Work out the finished part from the listing and answer in its coordinate system (mm). A direction names the side the tool comes from. Give positions to 0.01 mm unless a question says otherwise; leave off trailing zeros. Write each loop counter-clockwise with the first axis right and the second up, starting at its lowest first coordinate (ties: lowest second). Pieces come first, ordered by that corner, then holes. Notation, with made-up numbers: (30, 63.5) -> (65, 63.5) arc R19 ccw to (65, 92.5) -> close; hole circle Ø6 at (54.5, -26.75). An arc over 180 degrees is marked (long way). Use a Markdown table: item, result. Add a question column.
Q1. Each of these flat-tipped pins is pushed along its axis until it touches: pin 1 Ø6.5 at (x, y) = (-21, 3) entering from +Z; pin 2 Ø4 at (x, y) = (21.5, -10) entering from +Z (3 decimals). Where does it stop, or does it pass through?
Q2. Section B-B, the plane y = 0 is taken. State how many separate pieces and enclosed holes the cut face has, plus the area to 3 significant figures.
Q3. Consider line 1 (X direction, y = 0, z = 1.35); line 2 (Y direction, x = -19.05, z = 1.5); line 3 (X direction, y = 1, z = 0.65). Determine where each line is inside the solid, lowest interval first.
Q4. For faces 1 (the face through (27, 0, 1.905)), 2 (the face through (23, -3, 1.651)), 3 (the face through (-27, 0, 1.905)), determine the directions among +Z, -Z, +X, -X, +Y, -Y from which every point of the face is accessible in a straight line to the end or side of a thin tool.
Q5. Section D-D, the plane x = -27 is taken. Give the vertices of the cut face in (y, z) (3 decimals).
Q6. For a pull along Y with two mould halves and no side action, classify faces 4 (the face through (-1, 0, 0)), 5 (the face through (-14.5, 1.4, 1.3)), 6 (the face through (-1, -12.7, 1)) as pulls with the +Y half, pulls with the -Y half, needs draft (parallel to the pull), parting line crosses it, or undercut.
from build123d import *

# Parameters (mm, degrees)
SKETCH_W        = 76.2
SKETCH_H        = 25.4
SKETCH_R        = 4.7625
PAD_DEPTH       = 1.905
SKETCH001_W     = 12.7
SKETCH001_H     = 12.7
POCKET_DEPTH    = 0.254
CHAMFER_SIZE    = 1
FILLET_R        = 1
SKETCH002_W     = 20.32
SKETCH002_H     = 25.4
PAD001_DEPTH    = 0.9525
CHAMFER001_SIZE = 0.9144


with BuildPart() as part:
    # Sketch → Pad (new body)
    with BuildSketch(Plane.XY):
        Rectangle(SKETCH_W, SKETCH_H)
        with Locations((-19.05, 0)):
            Circle(SKETCH_R, mode=Mode.SUBTRACT)
        with Locations((19.05, 0)):
            Circle(SKETCH_R, mode=Mode.SUBTRACT)
    extrude(amount=PAD_DEPTH)

    # Sketch001 → Pocket (cut)
    with BuildSketch(Plane.XY.offset(1.905)):
        with Locations((-19.05, 0)):
            Rectangle(SKETCH001_W, SKETCH001_H)
        with Locations((19.05, 0)):
            Rectangle(SKETCH001_W, SKETCH001_H)
    extrude(amount=-POCKET_DEPTH, mode=Mode.SUBTRACT)

    # Chamfer
    chamfer_edges = [part.edges().sort_by_distance(p)[0] for p in [
        (14.2875, 0, 0),
        (-23.8125, 0, 0),
    ]]
    chamfer(chamfer_edges, length=CHAMFER_SIZE)

    # Fillet
    fillet_edges = [part.edges().sort_by_distance(p)[0] for p in [
        (38.1, 12.7, 0.9525),
        (38.1, -12.7, 0.9525),
        (-38.1, -12.7, 0.9525),
        (-38.1, 12.7, 0.9525),
    ]]
    fillet(fillet_edges, radius=FILLET_R)

    # Sketch002 (on Face5 of Pocket) → Pad001 (join)
    with BuildSketch(Plane.XY.offset(1.905)):
        Rectangle(SKETCH002_W, SKETCH002_H)
    extrude(amount=PAD001_DEPTH)

    # Chamfer001
    chamfer001_edges = [part.edges().sort_by_distance(p)[0] for p in [
        (0, -12.7, 2.8575),
        (-10.16, 0, 2.8575),
        (0, 12.7, 2.8575),
        (10.16, 0, 2.8575),
    ]]
    chamfer(chamfer001_edges, length=CHAMFER001_SIZE)


solid = part.part
Result set:
| question | item | result |
|---|---|---|
| 1 | pin 1 | stops at z = 1.65 |
| 1 | pin 2 | stops at z = 1.905 |
| 2 | separate pieces | 3 |
| 2 | enclosed holes | 0 |
| 2 | area | 124 mm2 |
| 3 | line 1 | x = -38.1 to -23.81, -14.29 to 14.29, 23.81 to 38.1 |
| 3 | line 2 | y = -12.7 to -4.76, 4.76 to 12.7 |
| 3 | line 3 | x = -38.1 to -24.06, -14.04 to 14.04, 24.06 to 38.1 |
| 4 | face 1 | +Z, +X, +Y, -Y |
| 4 | face 2 | +Z |
| 4 | face 3 | +Z, -X, +Y, -Y |
| 5 | outline | (-12.7, 0) -> (12.7, 0) -> (12.7, 1.905) -> (-12.7, 1.905) -> close |
| 6 | face 4 | needs draft |
| 6 | face 5 | undercut |
| 6 | face 6 | pulls with the -Y half |
